Geometry: final body of the model. Coordinates: model frame, mm. A direction names the side the tool comes from. Give positions to 0.01 mm unless a question says otherwise; leave off trailing zeros. Order: outer loops, then holes, each group sorted by start corner. A loop starts at its lowest first (then second) coordinate and runs counter-clockwise, first axis right, second up. Notation, with made-up numbers: (82, 32.5) - (110, 32.5) arc R21 cw to (110, 55.5) - close; hole circle Ø10 at (19, 24.5). An arc over 180 degrees is marked (long way). One line per item, written item: value.
```python
from build123d import *

# Parameters (mm, degrees)
BASE_FLANGE1_DEPTH               = 1371.6
F_17_64_0_26563_DIAMETER_HOLE1_D = 6.747002
SKETCH8_W                        = 28.575
SKETCH8_H                        = 69.85
CUT_EXTRUDE1_DEPTH               = 1374.480192795
F_10_0_1935_DIAMETER_HOLE1_D     = 4.9149
F_17_64_0_26563_DIAMETER_HOLE2_D = 6.747002
F_11_32_0_34375_DIAMETER_HOLE1_D = 8.73125
FILLET1_R                        = 3.175
CUT_EXTRUDE2_DEPTH               = 1374.480192795


# Sheet-metal steps are written as plain solids
with BuildPart() as part:
    # Sketch1 → Base-Flange1 (new body)
    with BuildSketch(Plane(origin=(0, 0, 0), x_dir=(1, 0, 0), z_dir=(0, 1, 0))):
        with BuildLine():
            Line((0, 50.8), (0, 6.35))
            ThreePointArc((0, 6.35), (1.859871939, 1.859871939), (6.35, 0))
            Line((6.35, 0), (50.8, 0))
            Line((50.8, 0), (50.8, 3.175))
            Line((50.8, 3.175), (6.35, 3.175))
            ThreePointArc((6.35, 3.175), (4.10493597, 4.10493597), (3.175, 6.35))
            Line((3.175, 6.35), (3.175, 50.8))
            Line((3.175, 50.8), (0, 50.8))
        make_face()
    extrude(amount=BASE_FLANGE1_DEPTH)

    # 17/64 (0.26563) Diameter Hole1 (through all)
    with Locations(Plane.ZY):
        with Locations((-38.1, 50.8), (-38.1, 685.8), (-38.1, 1320.8)):
            Hole(F_17_64_0_26563_DIAMETER_HOLE1_D / 2)

    # Sketch8 → Cut-Extrude1 (cut, through all)
    with BuildSketch(Plane.ZY):
        with Locations((-36.5125, 428.625)):
            Rectangle(SKETCH8_W, SKETCH8_H)
        with Locations((-36.5125, 942.975)):
            Rectangle(SKETCH8_W, SKETCH8_H)
    extrude(amount=-CUT_EXTRUDE1_DEPTH, mode=Mode.SUBTRACT)

    # #10 (0.1935) Diameter Hole1 (through all)
    with Locations(Plane.XY):
        with Locations((30.1625, 46.0375), (30.1625, 198.4375), (30.1625, 350.8375), (30.1625, 503.2375), (30.1625, 655.6375)):
            f_10_0_1935_diameter_hole1 = Hole(F_10_0_1935_DIAMETER_HOLE1_D / 2)

    # 17/64 (0.26563) Diameter Hole2 (through all)
    with Locations(Plane.XY):
        with Locations((33.3375, 179.1335), (33.3375, 331.5335), (33.3375, 483.9335), (33.3375, 636.3335)):
            f_17_64_0_26563_diameter_hole2 = Hole(F_17_64_0_26563_DIAMETER_HOLE2_D / 2)

    # 11/32 (0.34375) Diameter Hole1 (through all)
    with Locations(Plane.XY):
        with Locations((38.1, 1352.55), (38.1, 772.16)):
            f_11_32_0_34375_diameter_hole1 = Hole(F_11_32_0_34375_DIAMETER_HOLE1_D / 2)

    # Fillet1
    fillet1_edges = [part.edges().sort_by_distance(p)[0] for p in [
        (50.8, 1371.6, -1.5875),
        (1.5875, 393.7, -50.8),
        (1.5875, 463.55, -50.8),
        (1.5875, 463.55, -22.225),
        (1.5875, 393.7, -22.225),
        (1.5875, 908.05, -22.225),
        (1.5875, 908.05, -50.8),
        (1.5875, 977.9, -50.8),
        (1.5875, 977.9, -22.225),
        (50.8, 0, -1.5875),
        (1.5875, 1371.6, -50.8),
        (1.5875, 0, -50.8),
    ]]
    fillet(fillet1_edges, radius=FILLET1_R)

    # Mirror1: #10 (0.1935) Diameter Hole1, 17/64 (0.26563) Diameter Hole2, 11/32 (0.34375) Diameter Hole1 across plane
    add(f_10_0_1935_diameter_hole1.mirror(Plane.ZX.offset(685.8)), mode=Mode.SUBTRACT)
    add(f_17_64_0_26563_diameter_hole2.mirror(Plane.ZX.offset(685.8)), mode=Mode.SUBTRACT)
    add(f_11_32_0_34375_diameter_hole1.mirror(Plane.ZX.offset(685.8)), mode=Mode.SUBTRACT)

    # Sketch15 → Cut-Extrude2 (cut, through all)
    with BuildSketch(Plane.ZY):
        with BuildLine():
            Line((-41.4734375, 1314.45), (-41.4734375, 1327.15))
            ThreePointArc((-41.4734375, 1327.15), (-38.1, 1330.5234375), (-34.7265625, 1327.15))
            Line((-34.7265625, 1327.15), (-34.7265625, 1314.45))
            ThreePointArc((-34.7265625, 1314.45), (-38.1, 1311.0765625), (-41.4734375, 1314.45))
        make_face()
        with BuildLine():
            Line((-41.4734375, 679.45), (-41.4734375, 692.15))
            ThreePointArc((-41.4734375, 692.15), (-38.1, 695.5234375), (-34.7265625, 692.15))
            Line((-34.7265625, 692.15), (-34.7265625, 679.45))
            ThreePointArc((-34.7265625, 679.45), (-38.1, 676.0765625), (-41.4734375, 679.45))
        make_face()
        with BuildLine():
            Line((-41.4734375, 44.45), (-41.4734375, 57.15))
            ThreePointArc((-41.4734375, 57.15), (-38.1, 60.5234375), (-34.7265625, 57.15))
            Line((-34.7265625, 57.15), (-34.7265625, 44.45))
            ThreePointArc((-34.7265625, 44.45), (-38.1, 41.0765625), (-41.4734375, 44.45))
        make_face()
    extrude(amount=-CUT_EXTRUDE2_DEPTH, mode=Mode.SUBTRACT)


solid = part.part
```
1) Section A-A, the plane y = 412.5. Return loops of the section in (x, z) (3 decimals).
Answers below:
outline: (0, -22.225) - (3.175, -22.225) - (3.175, -6.35) arc R3.175 cw to (6.35, -3.175) - (50.8, -3.175) - (50.8, 0) - (6.35, 0) arc R6.35 ccw to (0, -6.35) - close
2) Material intervals for line 1 along Z through (x, y) = (47, 1160.5) (3 decimals); line 2 along X through (y, z) = (1089, -13) (3 decimals); line 3 along X through (y, z) = (802.5, -2), sorted ascending.
Answers below:
line 1: -3.175 to 0
line 2: 0 to 3.175
line 3: 1.72 to 50.8
3) Section B-B, the plane y = 801. Return loops of the section in (x, z) (3 decimals).
Answers below:
outline: (0, -50.8) - (3.175, -50.8) - (3.175, -6.35) arc R3.175 cw to (6.35, -3.175) - (50.8, -3.175) - (50.8, 0) - (6.35, 0) arc R6.35 ccw to (0, -6.35) - close
4) Section C-C, the plane x = 14. Return loops of the section in (y, z) (3 decimals), then the cut area to 3 significant figures.
Answers below:
outline: (0, -3.175) - (1371.6, -3.175) - (1371.6, 0) - (0, 0) - close
area: 4,350 mm^2
5) Set-up query: faces 1 (the face through (3.175, 676, -28)), 2 (the face through (3, 0, -13)). Return all of +Z, -Z, +X, -X, +Y, -Y with unobstructed straight access to the full face (end or side cutting, diameter ignored); none if empty.
Answers below:
face 1: -Z, +X, +Y, -Y
face 2: +Z, -Z, +X, -X, -Y
6) First-contact query: pin 1 (5.5 mm diameter, centred on x = 30.16, y = 1325.56, fed in from -Z) (3 decimals); pin 2 (13.5 mm diameter, centred on y = 873.5, z = -39.5, fed in from +X) (3 decimals). Flat tips, straight axial feed; report the tip coordinate or a pass-through.
Answers below:
pin 1: z = -3.175
pin 2: x = 3.175
